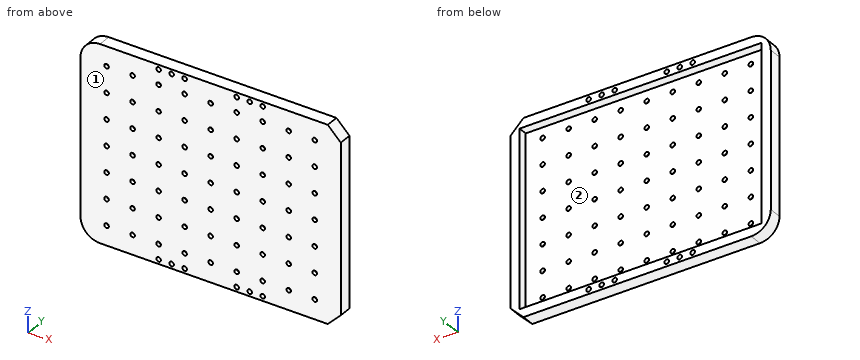
```python
from build123d import *

# Parameters (mm, degrees)
SKETCH1_W                   = 200
SKETCH1_H                   = 150
CHASIS_DEPTH                = 10
SKETCH2_W                   = 186
SKETCH2_H                   = 136
CHASIS_EDGE_DEPTH           = 7
HOLE_PATTERN_R              = 1.75
GENERAL_PURPOSE_HOLES_DEPTH = 251.0979808
SKETCH16_R                  = 1.75
CUT_EXTRUDE4_DEPTH          = 251.199920064
CHAMFER2_SIZE               = 10
FILLET2_R                   = 15


with BuildPart() as part:
    # Sketch1 → Chasis (new body)
    with BuildSketch(Plane(origin=(0, 0, 0), x_dir=(1, 0, 0), z_dir=(0, 1, 0))):
        with Locations((100, 75)):
            Rectangle(SKETCH1_W, SKETCH1_H)
    extrude(amount=CHASIS_DEPTH)

    # Sketch2 → Chasis Edge (cut)
    with BuildSketch(Plane(origin=(0, 10, 0), x_dir=(1, 0, 0), z_dir=(0, 1, 0))):
        with Locations((100, 75)):
            Rectangle(SKETCH2_W, SKETCH2_H)
    extrude(amount=-CHASIS_EDGE_DEPTH, mode=Mode.SUBTRACT)

    # Hole Pattern → General Purpose Holes (cut, through all)
    with BuildSketch(Plane(origin=(0, 3, 0), x_dir=(1, 0, 0), z_dir=(0, 1, 0))):
        with Locations(Location((20, 135, 0), (0, 0, 270))):
            Circle(HOLE_PATTERN_R)
        with Locations(Location((40, 135, 0), (0, 0, 270))):
            Circle(HOLE_PATTERN_R)
        with Locations(Location((60, 135, 0), (0, 0, 270))):
            Circle(HOLE_PATTERN_R)
        with Locations(Location((80, 135, 0), (0, 0, 270))):
            Circle(HOLE_PATTERN_R)
        with Locations(Location((100, 135, 0), (0, 0, 270))):
            Circle(HOLE_PATTERN_R)
        with Locations(Location((120, 135, 0), (0, 0, 270))):
            Circle(HOLE_PATTERN_R)
        with Locations(Location((140, 135, 0), (0, 0, 270))):
            Circle(HOLE_PATTERN_R)
        with Locations(Location((160, 135, 0), (0, 0, 270))):
            Circle(HOLE_PATTERN_R)
        with Locations(Location((180, 135, 0), (0, 0, 270))):
            Circle(HOLE_PATTERN_R)
        with Locations(Location((20, 115, 0), (0, 0, 270))):
            Circle(HOLE_PATTERN_R)
        with Locations(Location((40, 115, 0), (0, 0, 270))):
            Circle(HOLE_PATTERN_R)
        with Locations(Location((60, 115, 0), (0, 0, 270))):
            Circle(HOLE_PATTERN_R)
        with Locations(Location((80, 115, 0), (0, 0, 270))):
            Circle(HOLE_PATTERN_R)
        with Locations(Location((100, 115, 0), (0, 0, 270))):
            Circle(HOLE_PATTERN_R)
        with Locations(Location((120, 115, 0), (0, 0, 270))):
            Circle(HOLE_PATTERN_R)
        with Locations(Location((140, 115, 0), (0, 0, 270))):
            Circle(HOLE_PATTERN_R)
        with Locations(Location((160, 115, 0), (0, 0, 270))):
            Circle(HOLE_PATTERN_R)
        with Locations(Location((180, 115, 0), (0, 0, 270))):
            Circle(HOLE_PATTERN_R)
        with Locations(Location((20, 95, 0), (0, 0, 270))):
            Circle(HOLE_PATTERN_R)
        with Locations(Location((40, 95, 0), (0, 0, 270))):
            Circle(HOLE_PATTERN_R)
        with Locations(Location((60, 95, 0), (0, 0, 270))):
            Circle(HOLE_PATTERN_R)
        with Locations(Location((80, 95, 0), (0, 0, 270))):
            Circle(HOLE_PATTERN_R)
        with Locations(Location((100, 95, 0), (0, 0, 270))):
            Circle(HOLE_PATTERN_R)
        with Locations(Location((120, 95, 0), (0, 0, 270))):
            Circle(HOLE_PATTERN_R)
        with Locations(Location((140, 95, 0), (0, 0, 270))):
            Circle(HOLE_PATTERN_R)
        with Locations(Location((160, 95, 0), (0, 0, 270))):
            Circle(HOLE_PATTERN_R)
        with Locations(Location((180, 95, 0), (0, 0, 270))):
            Circle(HOLE_PATTERN_R)
        with Locations(Location((20, 75, 0), (0, 0, 270))):
            Circle(HOLE_PATTERN_R)
        with Locations(Location((40, 75, 0), (0, 0, 270))):
            Circle(HOLE_PATTERN_R)
        with Locations(Location((60, 75, 0), (0, 0, 270))):
            Circle(HOLE_PATTERN_R)
        with Locations(Location((80, 75, 0), (0, 0, 270))):
            Circle(HOLE_PATTERN_R)
        with Locations(Location((100, 75, 0), (0, 0, 270))):
            Circle(HOLE_PATTERN_R)
        with Locations(Location((120, 75, 0), (0, 0, 270))):
            Circle(HOLE_PATTERN_R)
        with Locations(Location((140, 75, 0), (0, 0, 270))):
            Circle(HOLE_PATTERN_R)
        with Locations(Location((160, 75, 0), (0, 0, 270))):
            Circle(HOLE_PATTERN_R)
        with Locations(Location((180, 75, 0), (0, 0, 270))):
            Circle(HOLE_PATTERN_R)
        with Locations(Location((20, 55, 0), (0, 0, 270))):
            Circle(HOLE_PATTERN_R)
        with Locations(Location((40, 55, 0), (0, 0, 270))):
            Circle(HOLE_PATTERN_R)
        with Locations(Location((60, 55, 0), (0, 0, 270))):
            Circle(HOLE_PATTERN_R)
        with Locations(Location((80, 55, 0), (0, 0, 270))):
            Circle(HOLE_PATTERN_R)
        with Locations(Location((100, 55, 0), (0, 0, 270))):
            Circle(HOLE_PATTERN_R)
        with Locations(Location((120, 55, 0), (0, 0, 270))):
            Circle(HOLE_PATTERN_R)
        with Locations(Location((140, 55, 0), (0, 0, 270))):
            Circle(HOLE_PATTERN_R)
        with Locations(Location((160, 55, 0), (0, 0, 270))):
            Circle(HOLE_PATTERN_R)
        with Locations(Location((180, 55, 0), (0, 0, 270))):
            Circle(HOLE_PATTERN_R)
        with Locations(Location((20, 35, 0), (0, 0, 270))):
            Circle(HOLE_PATTERN_R)
        with Locations(Location((40, 35, 0), (0, 0, 270))):
            Circle(HOLE_PATTERN_R)
        with Locations(Location((60, 35, 0), (0, 0, 270))):
            Circle(HOLE_PATTERN_R)
        with Locations(Location((80, 35, 0), (0, 0, 270))):
            Circle(HOLE_PATTERN_R)
        with Locations(Location((100, 35, 0), (0, 0, 270))):
            Circle(HOLE_PATTERN_R)
        with Locations(Location((120, 35, 0), (0, 0, 270))):
            Circle(HOLE_PATTERN_R)
        with Locations(Location((140, 35, 0), (0, 0, 270))):
            Circle(HOLE_PATTERN_R)
        with Locations(Location((160, 35, 0), (0, 0, 270))):
            Circle(HOLE_PATTERN_R)
        with Locations(Location((180, 35, 0), (0, 0, 270))):
            Circle(HOLE_PATTERN_R)
        with Locations(Location((20, 15, 0), (0, 0, 270))):
            Circle(HOLE_PATTERN_R)
        with Locations(Location((40, 15, 0), (0, 0, 270))):
            Circle(HOLE_PATTERN_R)
        with Locations(Location((60, 15, 0), (0, 0, 270))):
            Circle(HOLE_PATTERN_R)
        with Locations(Location((80, 15, 0), (0, 0, 270))):
            Circle(HOLE_PATTERN_R)
        with Locations(Location((100, 15, 0), (0, 0, 270))):
            Circle(HOLE_PATTERN_R)
        with Locations(Location((120, 15, 0), (0, 0, 270))):
            Circle(HOLE_PATTERN_R)
        with Locations(Location((140, 15, 0), (0, 0, 270))):
            Circle(HOLE_PATTERN_R)
        with Locations(Location((160, 15, 0), (0, 0, 270))):
            Circle(HOLE_PATTERN_R)
        with Locations(Location((180, 15, 0), (0, 0, 270))):
            Circle(HOLE_PATTERN_R)
    extrude(amount=-GENERAL_PURPOSE_HOLES_DEPTH, mode=Mode.SUBTRACT)

    # Sketch16 → Cut-Extrude4 (cut, through all)
    with BuildSketch(Plane(origin=(0, 10, 0), x_dir=(1, 0, 0), z_dir=(0, 1, 0))):
        with Locations(Location((130, 146.5, 0), (0, 0, 270))):
            Circle(SKETCH16_R)
        with Locations(Location((120, 146.5, 0), (0, 0, 270))):
            Circle(SKETCH16_R)
        with Locations(Location((140, 146.5, 0), (0, 0, 270))):
            Circle(SKETCH16_R)
        with Locations(Location((140, 3.5, 0), (0, 0, 90))):
            Circle(SKETCH16_R)
        with Locations(Location((120, 3.5, 0), (0, 0, 90))):
            Circle(SKETCH16_R)
        with Locations(Location((130, 3.5, 0), (0, 0, 90))):
            Circle(SKETCH16_R)
        with Locations(Location((70, 3.5, 0), (0, 0, 270))):
            Circle(SKETCH16_R)
        with Locations(Location((80, 3.5, 0), (0, 0, 270))):
            Circle(SKETCH16_R)
        with Locations(Location((60, 3.5, 0), (0, 0, 270))):
            Circle(SKETCH16_R)
        with Locations(Location((60, 146.5, 0), (0, 0, 90))):
            Circle(SKETCH16_R)
        with Locations(Location((80, 146.5, 0), (0, 0, 90))):
            Circle(SKETCH16_R)
        with Locations(Location((70, 146.5, 0), (0, 0, 90))):
            Circle(SKETCH16_R)
    extrude(amount=-CUT_EXTRUDE4_DEPTH, mode=Mode.SUBTRACT)

    # Chamfer2
    chamfer2_edges = [part.edges().sort_by_distance(p)[0] for p in [
        (200, 5, -150),
        (200, 5, 0),
    ]]
    chamfer(chamfer2_edges, length=CHAMFER2_SIZE)

    # Fillet2
    fillet2_edges = [part.edges().sort_by_distance(p)[0] for p in [
        (0, 5, -150),
        (0, 5, 0),
    ]]
    fillet(fillet2_edges, radius=FILLET2_R)


solid = part.part
```
CAD build for the part. Positions are in the model's coordinates, mm. Face numbers are marked on the shaded views. Give positions to 0.01 mm unless a question says otherwise; leave off trailing zeros. Order: outer loops, then holes, each group sorted by start corner. A loop starts at its lowest first (then second) coordinate and runs counter-clockwise, first axis right, second up.
(1) Drill centre lines: L1, parallel to Z at x = 101, y = 4.5; L2, parallel to X at y = 6.75, z = -78.5; L3, parallel to Z at x = 61, y = 6. Where is each one in solid material? Low to high.
(2) Mould opens along Z. For the marked faces 1 and 2 say: released by +Z, released by -Z, zero draft, split by the parting line, or undercut.
(3) Saw through at B-B, the plane z = -127.5. Give the cut face in (x, y), then the cut area to 3 significant figures.
(4) Saw through at A-A, the plane y = 8. State how many separate pieces and enclosed holes the cut face has, then the cut area to 3 significant figures.
(5) Saw through at C-C, the plane x = 187.5. Give the cut face in (y, z).
(6) Flat gauge pin, fed straight in: pin 1 (4.5 mm diameter, centred on x = 160, z = -55, fed in from +Y). Where does the tip first touch, or does it go through?
Results found:
1. L1: z = -150 to -143, -7 to 0
1. L2: x = 0 to 7, 193 to 200
1. L3: z = -150 to -147.94, -145.06 to -143, -7 to -4.94, -2.06 to 0
2. face 1: zero draft
2. face 2: undercut
3. outline: (0, 0) - (200, 0) - (200, 10) - (193, 10) - (193, 3) - (7, 3) - (7, 10) - (0, 10) - close
3. area: 698 mm2
4. separate pieces: 1
4. enclosed holes: 13
4. area: 4,390 mm2
5. outline: (0, -150) - (10, -150) - (10, -143) - (3, -143) - (3, -7) - (10, -7) - (10, 0) - (0, 0) - close
6. pin 1: stops at y = 3
